Source: three-view drawing plus pictorial views. Frame: mm from the lowest corner of the part. A direction names the side the tool comes from. Give positions to 0.01 mm unless a question says otherwise; leave off trailing zeros. Loops run counter-clockwise (first coordinate to the right, second up) from the corner with the lowest first, then second, coordinate; pieces in that order, holes last. Notation, with made-up numbers: M 36,87.5 L 92,87.5 A10 ccw 92,102.5 Z; hole C -1,1.25 d2. An arc over 180 degrees is marked long. Write item = value, one per line.
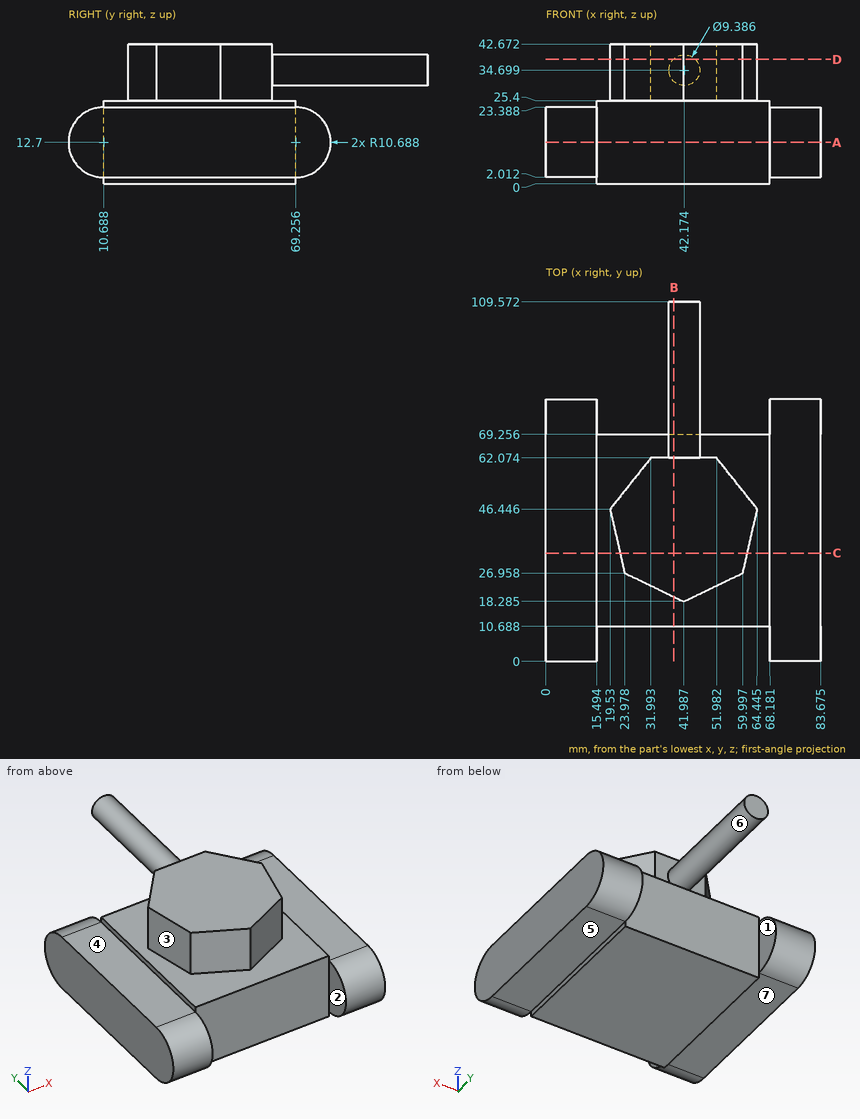
1. Reachability of the marked faces 5, 6 and 7 from +Z, -Z, +X, -X, +Y, -Y: full face, straight path, thin tool, end or side. Return the list, or none.
Derived:
face_5 = -Z, +X, +Y, -Y
face_6 = +Y
face_7 = -Z, -X, +Y, -Y
2. Pull-direction query (X, two-part tool) for the marked faces 1, 2, 3 and 4; classes: +X half, -X half, draft (parallel to the pull), parting line (faces both ways), or undercut.
Derived:
face_1 = undercut
face_2 = undercut
face_3 = -X half
face_4 = draft
3. Cut plane C-C, the plane y = 33. Return the cut outline in (x, z) (1 decimal).
Derived:
outline = M 0,2 L 15.5,2 L 15.5,0 L 68.2,0 L 68.2,2 L 83.7,2 L 83.7,23.4 L 68.2,23.4 L 68.2,25.4 L 61.4,25.4 L 61.4,42.7 L 22.6,42.7 L 22.6,25.4 L 15.5,25.4 L 15.5,23.4 L 0,23.4 Z
4. First-contact query: pin 1 Ø12 at (x, z) = (31, 36) entering from +Y; pin 2 Ø6 at (x, z) = (72, 8.5) entering from +Y; pin 3 Ø4.5 at (x, y) = (6.5, 31) entering from +Z. Flat tips, straight axial feed; report the tip coordinate or a pass-through.
Derived:
pin_1 = 62.07
pin_2 = 79.88
pin_3 = 23.39
5. Material intervals for probe 1 along Z at (x, y) = (25, 62.5); probe 2 along Y at (x, z) = (34, 2.5) (1 decimal); probe 3 along X at (y, z) = (52, 40) (1 decimal), sorted ascending. Write a range as from..to.
Derived:
probe_1 = 0..25.4
probe_2 = 10.7..69.3
probe_3 = 24..60
6. Cut plane B-B, the plane x = 39. Return the cut outline in (y, z) (1 decimal).
Derived:
outline = M 10.7,0 L 69.3,0 L 69.3,25.4 L 62.1,25.4 L 62.1,31.2 L 109.6,31.2 L 109.6,38.2 L 62.1,38.2 L 62.1,42.7 L 19.7,42.7 L 19.7,25.4 L 10.7,25.4 Z
7. Cut plane D-D, the plane z = 38. Return the cut outline in (x, y) (1 decimal), then the cut area to 3 significant figures.
Derived:
outline = M 19.5,46.4 L 24,27 L 42,18.3 L 60,27 L 64.4,46.4 L 52,62.1 L 45.5,62.1 L 45.5,109.6 L 38.8,109.6 L 38.8,62.1 L 32,62.1 Z
area = 1,770 mm²
8. Cut plane A-A, the plane z = 12.7. Return the cut outline in (x, y) (1 decimal).
Derived:
outline = M 0,0 L 15.5,0 L 15.5,10.7 L 68.2,10.7 L 68.2,0 L 83.7,0 L 83.7,79.9 L 68.2,79.9 L 68.2,69.3 L 15.5,69.3 L 15.5,79.9 L 0,79.9 Z
